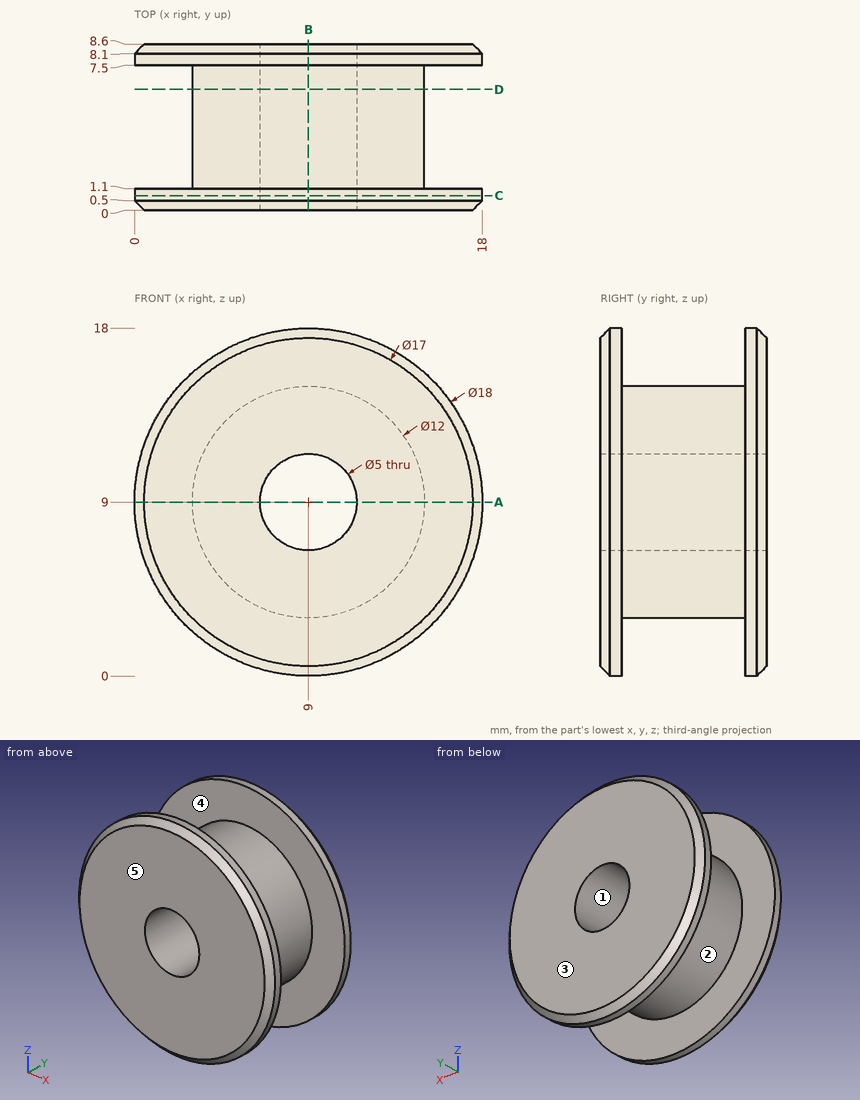
Design review of the part shown in the three views and the two pictorial views. Dimensions are in mm from the part's minimum x, y and z. A direction names the side the tool comes from. Round coordinates to 2 decimals unless told otherwise and drop trailing zeros. Write each loop counter-clockwise with the first axis right and the second up, starting at its lowest first coordinate (ties: lowest second). Pieces come first, ordered by that corner, then holes.
Item 1: Consider section D-D on y = 6.25. Give the boundary of the cut face in (x, z), and give its area (3 significant figures).
Item 2: For the marked faces 1 and 2, list the 3-axis set-ups (+Z, -Z, +X, -X, +Y, -Y) from which the entire face can be reached by the end or side of a thin tool; tool diameter is ignored.
Item 3: Consider section A-A on z = 9. Give the boundary of the cut face in (x, y).
Item 4: Consider section C-C on y = 0.75. Give the boundary of the cut face in (x, z), and give its area (3 significant figures).
Item 5: Draft analysis for pull direction Y (two halves, no side actions). For the marked faces 3, 4 and 5, state which applies: released by +Y, released by -Y, zero draft, split by the parting line, or undercut.
Item 6: Wall thickness on L1, parallel to Y at x = 4, z = 5; L2, parallel to Z at x = 9, y = 4.75: over which ranges is each line inside the solid? List them lowest first.
Item 7: For pin 1 Ø5 at (x, y) = (14, 1.5) entering from +Z; pin 2 Ø4.5 at (x, z) = (9, 9) entering from +Y; pin 3 Ø1 at (x, y) = (13.5, 2) entering from -Z; pin 4 Ø3 at (y, z) = (1.5, 7) entering from +X, all flat-tipped, find the tip position at first contact; note any pin that passes through.
Item 8: Consider section B-B on x = 9. Give the boundary of the cut face in (y, z).
Check values:
1. outline: circle Ø12 at (9, 9); hole circle Ø5 at (9, 9)
1. area: 93.5 mm2
2. face 1: +Y, -Y
2. face 2: none
3. outline: (0, 0.5) - (0.5, 0) - (6.5, 0) - (6.5, 8.6) - (0.5, 8.6) - (0, 8.1) - (0, 7.5) - (3, 7.5) - (3, 1.1) - (0, 1.1) - close; (11.5, 0) - (17.5, 0) - (18, 0.5) - (18, 1.1) - (15, 1.1) - (15, 7.5) - (18, 7.5) - (18, 8.1) - (17.5, 8.6) - (11.5, 8.6) - close
4. outline: circle Ø18 at (9, 9); hole circle Ø5 at (9, 9)
4. area: 235 mm2
5. face 3: released by +Y
5. face 4: undercut
5. face 5: released by -Y
6. L1: y = 0 to 1.1, 7.5 to 8.6
6. L2: z = 3 to 6.5, 11.5 to 15
7. pin 1: stops at z = 17.64
7. pin 2: passes through
7. pin 3: stops at z = 4.53
7. pin 4: stops at x = 17.98
8. outline: (0, 0.5) - (0.5, 0) - (1.1, 0) - (1.1, 3) - (7.5, 3) - (7.5, 0) - (8.1, 0) - (8.6, 0.5) - (8.6, 6.5) - (0, 6.5) - close; (0, 11.5) - (8.6, 11.5) - (8.6, 17.5) - (8.1, 18) - (7.5, 18) - (7.5, 15) - (1.1, 15) - (1.1, 18) - (0.5, 18) - (0, 17.5) - close
